Geometry check sheet. Reference: the model listing, model coordinates, mm. Face numbers are marked on the shaded views. A direction names the side the tool comes from. Coordinates: 2 decimals unless noted, no trailing zeros. Loops run counter-clockwise (first coordinate to the right, second up) from the corner with the lowest first, then second, coordinate; pieces in that order, holes last.
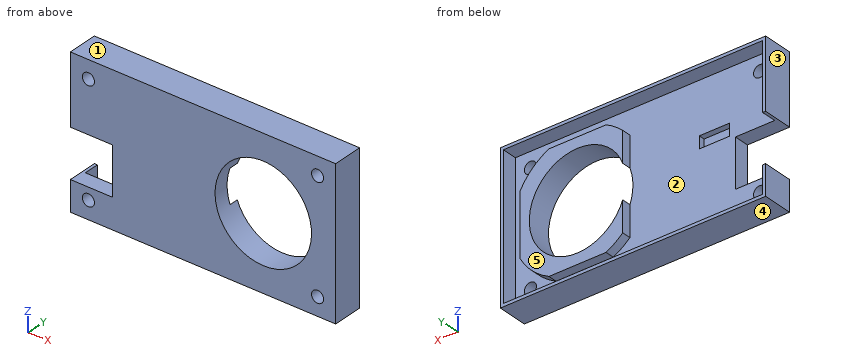
from build123d import *

# Parameters (mm, degrees)
SKETCH1_W           = 88
SKETCH1_H           = 49
BOSS_EXTRUDE1_DEPTH = 5
SKETCH2_W           = 88
SKETCH2_H           = 49
SKETCH2_W_2         = 86
SKETCH2_H_2         = 47
BOSS_EXTRUDE2_DEPTH = 5
SKETCH3_R           = 16
CUT_EXTRUDE1_DEPTH  = 5
CUT_EXTRUDE2_START  = -10
SKETCH4_W           = 14
SKETCH4_H           = 16
CUT_EXTRUDE2_DEPTH  = 10
SKETCH5_W           = 10
SKETCH5_H           = 4
CUT_EXTRUDE3_DEPTH  = 2
SKETCH6_R           = 21.682235108
SKETCH6_R_2         = 16
BOSS_EXTRUDE3_DEPTH = 3
SKETCH7_W           = 10
SKETCH7_H           = 35.531306717
CUT_EXTRUDE4_DEPTH  = 3
SKETCH8_R           = 2
CUT_EXTRUDE5_DEPTH  = 5
SKETCH9_W           = 40.675164953
SKETCH9_H           = 47
SKETCH9_W_2         = 34.982420928
SKETCH9_H_2         = 39
CUT_EXTRUDE6_DEPTH  = 3


with BuildPart() as part:
    # Sketch1 → Boss-Extrude1 (new body)
    with BuildSketch(Plane(origin=(0, 0, 0), x_dir=(1, 0, 0), z_dir=(0, 1, 0))):
        with Locations((44, 24.5)):
            Rectangle(SKETCH1_W, SKETCH1_H)
    extrude(amount=BOSS_EXTRUDE1_DEPTH)

    # Sketch2 → Boss-Extrude2 (add)
    with BuildSketch(Plane(origin=(0, 5, 0), x_dir=(1, 0, 0), z_dir=(0, 1, 0))):
        with Locations((44, 24.5)):
            Rectangle(SKETCH2_W, SKETCH2_H)
        with Locations((44, 24.5)):
            Rectangle(SKETCH2_W_2, SKETCH2_H_2, mode=Mode.SUBTRACT)
    extrude(amount=BOSS_EXTRUDE2_DEPTH)

    # Sketch3 → Cut-Extrude1 (cut)
    with BuildSketch(Plane(origin=(0, 0, 0), x_dir=(-1, 0, 0), z_dir=(0, -1, 0))):
        with Locations(Location((-64, 24.5, 0), (0, 0, 90))):
            Circle(SKETCH3_R)
    extrude(amount=-CUT_EXTRUDE1_DEPTH, mode=Mode.SUBTRACT)

    # Sketch4 → Cut-Extrude2 (cut)
    with BuildSketch(Plane.XZ.offset(CUT_EXTRUDE2_START)):
        with Locations((7, -31)):
            Rectangle(SKETCH4_W, SKETCH4_H)
    extrude(amount=CUT_EXTRUDE2_DEPTH, mode=Mode.SUBTRACT)

    # Sketch5 → Cut-Extrude3 (cut)
    with BuildSketch(Plane(origin=(0, 5, 0), x_dir=(1, 0, 0), z_dir=(0, 1, 0))):
        with Locations((21, 20)):
            Rectangle(SKETCH5_W, SKETCH5_H)
    extrude(amount=-CUT_EXTRUDE3_DEPTH, mode=Mode.SUBTRACT)

    # Sketch6 → Boss-Extrude3 (add)
    with BuildSketch(Plane(origin=(0, 5, 0), x_dir=(1, 0, 0), z_dir=(0, 1, 0))):
        with Locations(Location((64, 24.5, 0), (0, 0, 90))):
            Circle(SKETCH6_R)
        with Locations(Location((64, 24.5, 0), (0, 0, 90))):
            Circle(SKETCH6_R_2, mode=Mode.SUBTRACT)
    extrude(amount=BOSS_EXTRUDE3_DEPTH)

    # Sketch7 → Cut-Extrude4 (cut)
    with BuildSketch(Plane(origin=(0, 5, 0), x_dir=(1, 0, 0), z_dir=(0, 1, 0))):
        with Locations((44, 25.309726248)):
            Rectangle(SKETCH7_W, SKETCH7_H)
    extrude(amount=CUT_EXTRUDE4_DEPTH, mode=Mode.SUBTRACT)

    # Sketch8 → Cut-Extrude5 (cut)
    with BuildSketch(Plane(origin=(0, 0, 0), x_dir=(-1, 0, 0), z_dir=(0, -1, 0))):
        with Locations(Location((-82, 6, 0), (0, 0, 90))):
            Circle(SKETCH8_R)
        with Locations(Location((-6, 6, 0), (0, 0, 90))):
            Circle(SKETCH8_R)
        with Locations(Location((-6, 43, 0), (0, 0, 90))):
            Circle(SKETCH8_R)
        with Locations(Location((-82, 43, 0), (0, 0, 90))):
            Circle(SKETCH8_R)
    extrude(amount=-CUT_EXTRUDE5_DEPTH, mode=Mode.SUBTRACT)

    # Sketch9 → Cut-Extrude6 (cut)
    with BuildSketch(Plane(origin=(0, 5, 0), x_dir=(1, 0, 0), z_dir=(0, 1, 0))):
        with Locations((66.662417523, 24.5)):
            Rectangle(SKETCH9_W, SKETCH9_H)
        with Locations((65.508789536, 24.5)):
            Rectangle(SKETCH9_W_2, SKETCH9_H_2, mode=Mode.SUBTRACT)
    extrude(amount=CUT_EXTRUDE6_DEPTH, mode=Mode.SUBTRACT)


solid = part.part
(1) Scan lines: L1, parallel to X at y = 1.95, z = -6; L2, parallel to Z at x = 64, y = 5.5; L3, parallel to X at y = 9.5, z = -6. Record each from-to range of solid material in increasing order.
Findings:
L1: x = 0 to 4, 8 to 80, 84 to 88
L2: z = -49 to -48, -44 to -40.5, -8.5 to -5, -1 to 0
L3: x = 0 to 1, 87 to 88
(2) Access from +Z, -Z, +X, -X, +Y, -Y to the whole of each face (thin tool, end or side, straight path). Record for the marked faces 4 and 5.
Findings:
face 4: -Z, +X, -X, +Y, -Y
face 5: +Y
(3) Sectioned sample at D-D on x = 82. Record the cut outline in (y, z).
Findings:
outline: (0, -49) - (10, -49) - (10, -48) - (5, -48) - (5, -45) - (0, -45) - close; (0, -41) - (5, -41) - (5, -36.59) - (8, -36.59) - (8, -12.41) - (5, -12.41) - (5, -8) - (0, -8) - close; (0, -4) - (5, -4) - (5, -1) - (10, -1) - (10, 0) - (0, 0) - close
(4) Sectioned sample at A-A on x = 64. Record the cut outline in (y, z).
Findings:
outline: (0, -49) - (10, -49) - (10, -48) - (5, -48) - (5, -44) - (8, -44) - (8, -40.5) - (0, -40.5) - close; (0, -8.5) - (8, -8.5) - (8, -5) - (5, -5) - (5, -1) - (10, -1) - (10, 0) - (0, 0) - close
(5) Draft check along Z on the marked faces 1, 2 and 3. Enter one of: +Z half, -Z half, draft (parallel to the pull), parting line (faces both ways), or undercut.
Findings:
face 1: +Z half
face 2: undercut
face 3: draft
(6) Gauge pin test, flat ends, axial feed: pin 1 Ø4 at (y, z) = (8.5, -26) entering from -X; pin 2 Ø2.5 at (y, z) = (6, -33) entering from -X; pin 3 Ø1 at (x, z) = (22, -24) entering from +Y. Record the tip position at first contact, or that the pin passes through.
Findings:
pin 1: stops at x = 79.63
pin 2: stops at x = 14
pin 3: stops at y = 5
(7) Sectioned sample at C-C on y = 1.25. Record the cut outline in (x, z).
Findings:
outline: (0, -49) - (88, -49) - (88, 0) - (0, 0) - (0, -23) - (14, -23) - (14, -39) - (0, -39) - close; hole circle Ø4 at (6, -43); hole circle Ø4 at (6, -6); hole circle Ø32 at (64, -24.5); hole circle Ø4 at (82, -43); hole circle Ø4 at (82, -6)
(8) Sectioned sample at B-B on z = -24.5. Record the cut outline in (x, y).
Findings:
outline: (14, 0) - (48, 0) - (48, 5) - (14, 5) - close; (80, 0) - (88, 0) - (88, 10) - (87, 10) - (87, 5) - (83, 5) - (83, 8) - (80, 8) - close
